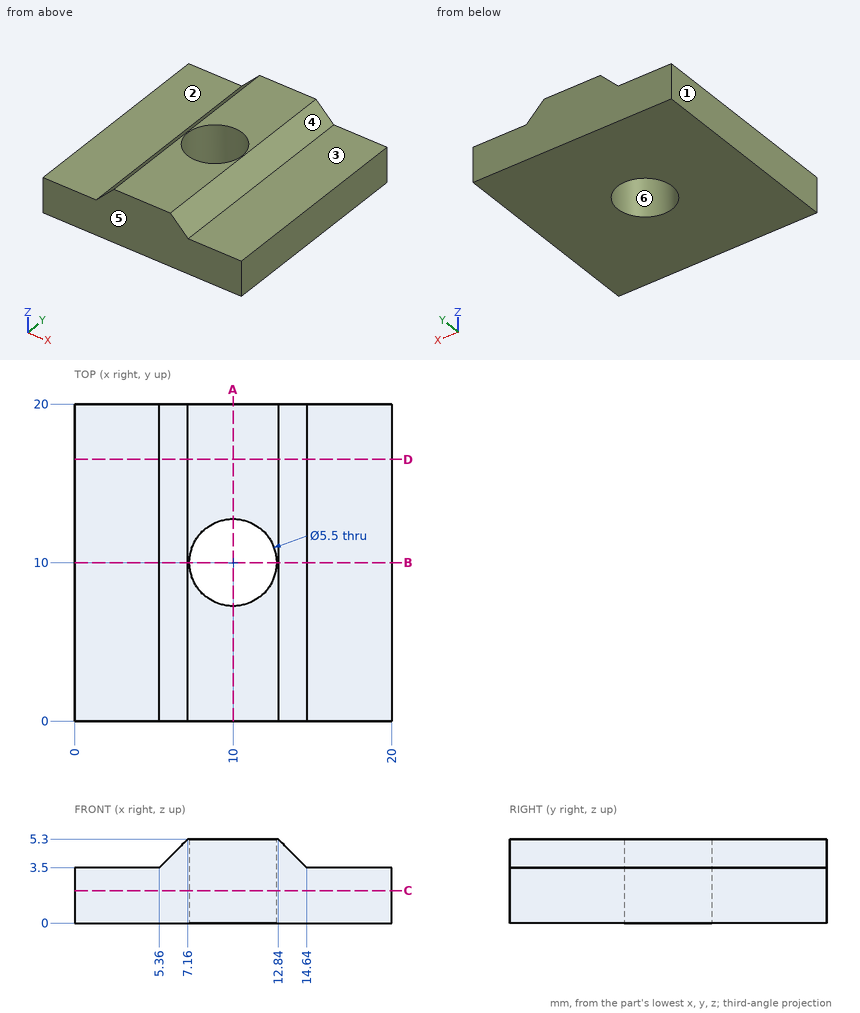
Geometry check sheet. Reference: drawing and pictorial views, mm from the part's lowest x, y, z. A direction names the side the tool comes from. Round coordinates to 2 decimals unless told otherwise and drop trailing zeros. Loops run counter-clockwise (first coordinate to the right, second up) from the corner with the lowest first, then second, coordinate; pieces in that order, holes last. Notation, with made-up numbers: (-28, 38.5) -> (-10, 38.5) arc R37 cw to (-10, 74.5) -> close; hole circle Ø1 at (47, -23.75). An arc over 180 degrees is marked (long way). Use a Markdown table: item, result.
(1) Go/stop test with flat-tipped pins: P1, Ø2, axis at x = 17, y = 5, coming from the +Z side; P2, Ø6, axis at x = 3, y = 13, coming from the +Z side. Record where each tip stops, or that it passes through.
Calculated:
| item | result |
|---|---|
| P1 | z = 3.5 |
| P2 | z = 4.14 |
(2) Sectioned sample at A-A (x = 10). Enter the section's corners in (y, z).
Calculated:
| item | result |
|---|---|
| outline | (0, 0) -> (7.25, 0) -> (7.25, 5.3) -> (0, 5.3) -> close; (12.75, 0) -> (20, 0) -> (20, 5.3) -> (12.75, 5.3) -> close |
(3) Sectioned sample at D-D (y = 16.5). Enter the section's corners in (x, z), then the cut area to 3 significant figures.
Calculated:
| item | result |
|---|---|
| outline | (0, 0) -> (20, 0) -> (20, 3.5) -> (14.64, 3.5) -> (12.84, 5.3) -> (7.16, 5.3) -> (5.36, 3.5) -> (0, 3.5) -> close |
| area | 83.5 mm² |
(4) Sectioned sample at C-C (z = 2.05). Enter the section's corners in (x, y).
Calculated:
| item | result |
|---|---|
| outline | (0, 0) -> (20, 0) -> (20, 20) -> (0, 20) -> close; hole circle Ø5.5 at (10, 10) |
(5) Scan lines: probe 1 along X at (y, z) = (10, 2.95); probe 2 along Z at (x, y) = (2, 13.25). Record each from-to range of solid material in increasing order.
Calculated:
| item | result |
|---|---|
| probe 1 | 0 to 7.25, 12.75 to 20 |
| probe 2 | 0 to 3.5 |
(6) Sectioned sample at B-B (y = 10). Enter the section's corners in (x, z), then the cut area to 3 significant figures.
Calculated:
| item | result |
|---|---|
| outline | (0, 0) -> (7.25, 0) -> (7.25, 5.3) -> (7.16, 5.3) -> (5.36, 3.5) -> (0, 3.5) -> close; (12.75, 0) -> (20, 0) -> (20, 3.5) -> (14.64, 3.5) -> (12.84, 5.3) -> (12.75, 5.3) -> close |
| area | 54.3 mm² |
(7) Set-up check for the marked faces 1, 2 and 3: record each of +Z, -Z, +X, -X, +Y, -Y from which the full face is reachable in a straight line by a thin tool's end or side.
Calculated:
| item | result |
|---|---|
| face 1 | +Z, -Z, -X, +Y, -Y |
| face 2 | +Z, -X, +Y, -Y |
| face 3 | +Z, +X, +Y, -Y |
(8) Mould release check, pull along X, two halves, no side actions. Record for the marked faces 4, 5 and 6: released by +X, released by -X, zero draft, split by the parting line, or undercut.
Calculated:
| item | result |
|---|---|
| face 4 | released by +X |
| face 5 | zero draft |
| face 6 | undercut |
